Work out the finished part from the listing and answer in its coordinate system (mm). A direction names the side the tool comes from. Coordinates: 2 decimals unless noted, no trailing zeros. Loops run counter-clockwise (first coordinate to the right, second up) from the corner with the lowest first, then second, coordinate; pieces in that order, holes last. Notation, with made-up numbers: (-10.75, 52) -> (21.25, 52) arc R27 cw to (21.25, 85) -> close; hole circle Ø9 at (79.5, -11). An arc over 180 degrees is marked (long way). Use a Markdown table: item, result.
from build123d import *

# Parameters (mm, degrees)
CROQUIS2_W              = 76.2
CROQUIS2_H              = 51
SALIENTE_EXTRUIR1_DEPTH = 433
CROQUIS6_W              = 70
CROQUIS6_H              = 44.8
CORTAR_EXTRUIR1_DEPTH   = 900
CROQUIS7_W              = 866
CROQUIS7_H              = 44.8
CORTAR_EXTRUIR2_DEPTH   = 20
CROQUIS8_R              = 6.5
CORTAR_EXTRUIR3_DEPTH   = 80


with BuildPart() as part:
    # Croquis2 → Saliente-Extruir1 (new, symmetric)
    with BuildSketch(Plane.XY):
        Rectangle(CROQUIS2_W, CROQUIS2_H)
    extrude(amount=SALIENTE_EXTRUIR1_DEPTH, both=True)

    # Croquis6 → Cortar-Extruir1 (cut)
    with BuildSketch(Plane.XY.offset(433)):
        Rectangle(CROQUIS6_W, CROQUIS6_H)
    extrude(amount=-CORTAR_EXTRUIR1_DEPTH, mode=Mode.SUBTRACT)

    # Croquis7 → Cortar-Extruir2 (cut)
    with BuildSketch(Plane.ZY.offset(38.1)):
        Rectangle(CROQUIS7_W, CROQUIS7_H)
    extrude(amount=-CORTAR_EXTRUIR2_DEPTH, mode=Mode.SUBTRACT)

    # Croquis8 → Cortar-Extruir3 (cut)
    with BuildSketch(Plane(origin=(0, 25.5, 0), x_dir=(1, 0, 0), z_dir=(0, 1, 0))):
        with Locations(Location((-8, 375, 0), (0, 0, 180))):
            Circle(CROQUIS8_R)
        with Locations(Location((-8, -375, 0), (0, 0, 180))):
            Circle(CROQUIS8_R)
    extrude(amount=-CORTAR_EXTRUIR3_DEPTH, mode=Mode.SUBTRACT)


solid = part.part
Q1. Determine the mould class of faces 3 (the flat face through (5, -23, 433)), 4 (the flat face through (-1, -25.5, 6)), 5 (the flat face through (-1, 25.5, 6)), 6 (the flat face through (-2, -22.4, -6)) for opening direction Y: pulls with the +Y half, pulls with the -Y half, needs draft (parallel to the pull), parting line crosses it, or undercut.
Solved:
| item | result |
|---|---|
| face 3 | needs draft |
| face 4 | pulls with the -Y half |
| face 5 | pulls with the +Y half |
| face 6 | undercut |
Q2. Given pin 1 Ø3 at (y, z) = (-1, 93.5) entering from -X, flat-ended and moving along its own axis, determine where the tip first touches the part or whether it passes through.
Solved:
| item | result |
|---|---|
| pin 1 | x = 35 |
Q3. Consider line 1 (Z direction, x = -8, y = -24.5); line 2 (X direction, y = -22.95, z = 375); line 3 (Y direction, x = 16, z = -158). Determine where each line is inside the solid, lowest interval first. Write a range as [from, to].
Solved:
| item | result |
|---|---|
| line 1 | [-433, -381.5], [-368.5, 368.5], [381.5, 433] |
| line 2 | [-38.1, -14.5], [-1.5, 38.1] |
| line 3 | [-25.5, -22.4], [22.4, 25.5] |
Q4. Section A-A on x = 27 is taken. Determine the outline of the cut face in (y, z).
Solved:
| item | result |
|---|---|
| outline | (-25.5, -433) -> (-22.4, -433) -> (-22.4, 433) -> (-25.5, 433) -> close; (22.4, -433) -> (25.5, -433) -> (25.5, 433) -> (22.4, 433) -> close |
Q5. For faces 1 (the flat face through (5, -23, -433)), 2 (the flat face through (35, 0, 6)), determine the directions among +Z, -Z, +X, -X, +Y, -Y from which every point of the face is accessible in a straight line to the end or side of a thin tool.
Solved:
| item | result |
|---|---|
| face 1 | -Z, +X, -X, +Y, -Y |
| face 2 | +Z, -Z, -X |
Q6. Section C-C on y = -6 is taken. Determine the outline of the cut face in (x, z).
Solved:
| item | result |
|---|---|
| outline | (35, -433) -> (38.1, -433) -> (38.1, 433) -> (35, 433) -> close |
Q7. Section B-B on z = -73 is taken. Determine the outline of the cut face in (x, y).
Solved:
| item | result |
|---|---|
| outline | (-38.1, -25.5) -> (38.1, -25.5) -> (38.1, 25.5) -> (-38.1, 25.5) -> (-38.1, 22.4) -> (35, 22.4) -> (35, -22.4) -> (-38.1, -22.4) -> close |
